from build123d import *

# Parameters (mm, degrees)
SKETCH_1_R               = 3.2
EXTRUDE_1_DEPTH          = 14
CUT_EXTRUDE_1_DEPTH      = 1
CUT_EXTRUDE_1_DEPTH_BACK = 10.4
SKETCH_3_W               = 0.65
SKETCH_3_H               = 3.2
CUT_EXTRUDE_2_DEPTH      = 1
SKETCH_4_W               = 0.4
SKETCH_4_H               = 2
EXTRUDE_2_DEPTH          = 4
EXTRUDE_2_2_DEPTH        = 4
SKETCH_4_W_2             = 2
SKETCH_4_H_2             = 0.4
EXTRUDE_2_3_DEPTH        = 4
EXTRUDE_3_DEPTH          = 2
EXTRUDE_4_DEPTH          = 2
SKETCH_8_R               = 3.2
SKETCH_8_R_2             = 0.603563731
EXTRUDE_5_DEPTH          = 2
SKETCH_9_R               = 0.5
CUT_EXTRUDE_3_DEPTH      = 10.8
SKETCH_10_R              = 0.5
CUT_EXTRUDE_4_DEPTH      = 2


with BuildPart() as part:
    # Sketch 1 → Extrude 1 (new body)
    with BuildSketch(Plane.XY):
        with BuildLine():
            Line((-4, 5.5), (4, 5.5))
            ThreePointArc((4, 5.5), (4.353553391, 5.353553391), (4.5, 5))
            Line((4.5, 5), (4.5, -5))
            ThreePointArc((4.5, -5), (4.353553391, -5.353553391), (4, -5.5))
            Line((4, -5.5), (-4, -5.5))
            ThreePointArc((-4, -5.5), (-4.353553391, -5.353553391), (-4.5, -5))
            Line((-4.5, -5), (-4.5, 5))
            ThreePointArc((-4.5, 5), (-4.353553391, 5.353553391), (-4, 5.5))
        make_face()
        with Locations((0, 1)):
            Circle(SKETCH_1_R, mode=Mode.SUBTRACT)
    extrude(amount=EXTRUDE_1_DEPTH)

    # Sketch 2 → Cut-Extrude 1 (cut, two sides)
    with BuildSketch(Plane.XY.offset(14)) as cut_extrude_1_sk:
        with BuildLine():
            ThreePointArc((-3.85, 1), (0, 4.85), (3.85, 1))
            Line((3.85, 1), (4.5, 1))
            Line((4.5, 1), (4.5, 5))
            ThreePointArc((4.5, 5), (4.353553391, 5.353553391), (4, 5.5))
            Line((4, 5.5), (-4, 5.5))
            ThreePointArc((-4, 5.5), (-4.353553391, 5.353553391), (-4.5, 5))
            Line((-4.5, 5), (-4.5, 1))
            Line((-4.5, 1), (-3.85, 1))
        make_face()
    extrude(amount=CUT_EXTRUDE_1_DEPTH, mode=Mode.SUBTRACT)
    extrude(cut_extrude_1_sk.sketch, amount=-CUT_EXTRUDE_1_DEPTH_BACK, mode=Mode.SUBTRACT)

    # Sketch 3 → Cut-Extrude 2 (cut)
    with BuildSketch(Plane.XY.offset(14)):
        with Locations((-4.175, -0.6)):
            Rectangle(SKETCH_3_W, SKETCH_3_H)
        with Locations((4.175, -0.6)):
            Rectangle(SKETCH_3_W, SKETCH_3_H)
    extrude(amount=-CUT_EXTRUDE_2_DEPTH, mode=Mode.SUBTRACT)



with BuildPart() as body_2:
    # Sketch 4 → Extrude 2 (new body)
    with BuildSketch(Plane(origin=(0, -5.5, 0), x_dir=(-1, 0, 0), z_dir=(0, -1, 0))):
        with Locations((4.7, -11)):
            Rectangle(SKETCH_4_W, SKETCH_4_H)
    extrude(amount=EXTRUDE_2_DEPTH)


with BuildPart() as body_3:
    # Sketch 4 → Extrude 2 2 (new body)
    with BuildSketch(Plane(origin=(0, -5.5, 0), x_dir=(-1, 0, 0), z_dir=(0, -1, 0))):
        with Locations((-4.7, -11)):
            Rectangle(SKETCH_4_W, SKETCH_4_H)
    extrude(amount=EXTRUDE_2_2_DEPTH)


with BuildPart() as body_4:
    # Sketch 4 → Extrude 2 3 (new body)
    with BuildSketch(Plane(origin=(0, -5.5, 0), x_dir=(-1, 0, 0), z_dir=(0, -1, 0))):
        with Locations((0, -13.7)):
            Rectangle(SKETCH_4_W_2, SKETCH_4_H_2)
    extrude(amount=EXTRUDE_2_3_DEPTH)


with BuildPart() as part_1:
    add(part.part)

    add(body_2.part)  # Extrude 3 merges body 2

    add(body_3.part)  # Extrude 3 merges body 3
    # Sketch 5 → Extrude 3 (add)
    with BuildSketch(Plane(origin=(0, 0, 10), x_dir=(-1, 0, 0), z_dir=(0, 0, -1))):
        with BuildLine():
            Line((4.5, -5.5), (4.5, -1.092241159))
            Line((4.5, -1.092241159), (4.6, -1.092241159))
            ThreePointArc((4.6, -1.092241159), (4.812132034, -1.180109124), (4.9, -1.392241159))
            Line((4.9, -1.392241159), (4.9, -5.5))
            Line((4.9, -5.5), (4.5, -5.5))
        make_face()
        with BuildLine():
            Line((-4.9, -1.392241159), (-4.9, -5.5))
            Line((-4.9, -5.5), (-4.5, -5.5))
            Line((-4.5, -5.5), (-4.5, -1.092241159))
            Line((-4.5, -1.092241159), (-4.6, -1.092241159))
            ThreePointArc((-4.6, -1.092241159), (-4.812132034, -1.180109124), (-4.9, -1.392241159))
        make_face()
    extrude(amount=-EXTRUDE_3_DEPTH)


    add(body_4.part)  # Extrude 4 merges body 4
    # Sketch 7 → Extrude 4 (add)
    with BuildSketch(Plane.ZY.offset(1)):
        with BuildLine():
            Line((14, -5.5), (14, 1))
            Line((14, 1), (13.6, 1))
            ThreePointArc((13.6, 1), (13.812132034, 0.912132034), (13.9, 0.7))
            Line((13.9, 0.7), (13.9, -5.5))
            Line((13.9, -5.5), (14, -5.5))
        make_face()
    extrude(amount=-EXTRUDE_4_DEPTH)

    # Sketch 8 → Extrude 5 (add)
    with BuildSketch(Plane.XY.offset(14)):
        with Locations((0, 1)):
            Circle(SKETCH_8_R)
        with Locations((0, 1)):
            Circle(SKETCH_8_R_2, mode=Mode.SUBTRACT)
    extrude(amount=-EXTRUDE_5_DEPTH)

    # Sketch 9 → Cut-Extrude 3 (cut, through all)
    with BuildSketch(Plane.ZY.offset(4.9)):
        with Locations((11, -8.5)):
            Circle(SKETCH_9_R)
        with BuildLine():
            Line((10, -8.5), (10, -9.805302044))
            Line((10, -9.805302044), (12, -9.805302044))
            Line((12, -9.805302044), (12, -8.5))
            ThreePointArc((12, -8.5), (11, -9.5), (10, -8.5))
        make_face()
    extrude(amount=-CUT_EXTRUDE_3_DEPTH, mode=Mode.SUBTRACT)

    # Sketch 10 → Cut-Extrude 4 (cut)
    with BuildSketch(Plane.XY.offset(13.9)):
        with Locations((0, -8.5)):
            Circle(SKETCH_10_R)
        with BuildLine():
            Line((-1, -8.5), (-1, -10.359825608))
            Line((-1, -10.359825608), (1, -10.359825608))
            Line((1, -10.359825608), (1, -8.5))
            ThreePointArc((1, -8.5), (0, -9.5), (-1, -8.5))
        make_face()
    extrude(amount=-CUT_EXTRUDE_4_DEPTH, mode=Mode.SUBTRACT)


solid = part_1.part
Here's how the part is built. I have some questions about the finished solid (model axes, mm). A direction names the side the tool comes from. Coordinates: 2 decimals unless noted, no trailing zeros. Loops run counter-clockwise (first coordinate to the right, second up) from the corner with the lowest first, then second, coordinate; pieces in that order, holes last. Notation, with made-up numbers: (69, 29) -> (73, 29) arc R21 ccw to (73, 51) -> close; hole circle Ø1 at (52.25, -32). An arc over 180 degrees is marked (long way). Use one line per item in the form item = value. Start each with the question number.
(1) Please list where these lines run through material, in increasing order: line 1 along X through (y, z) = (1, 13.15); line 2 along Y through (x, z) = (4.6, 11); line 3 along Z through (x, y) = (0, -0.25).
(2) Will these pins go through, and if not, where does the flat tip stop? pin 1 (0.5 mm diameter, centred on x = 4.5, z = 13.5, fed in from +Y); pin 2 (2 mm diameter, centred on x = 0.5, y = -7.5, fed in from +Z); pin 3 (2.5 mm diameter, centred on x = -1.5, z = 4, fed in from -Y).
(3) We'd pull the mould along Z, two halves only. Please class faces 5 (the face through (-4.703, -8.988, 10.892)), 6 (the face through (-0.08, 4.85, 8.87)), 7 (the face through (0, 0, 12)), 8 (the face through (4.697, -8.988, 10.892)): pulls with the +Z half, pulls with the -Z half, needs draft (parallel to the pull), parting line crosses it, or undercut.
(4) If we section it at C-C (z = 2.25): Please give me the cut outline in (x, y), then the cut area to 3 significant figures.
(5) On a 3-axis mill with a long thin cutter (end or side, diameter ignored), from which of +Z, -Z, +X, -X, +Y, -Y can I reach the whole of each face in a straight line? I mean faces 1 (the face through (0, -7, 13.5)), 2 (the face through (-3.85, -0.6, 13.5)), 3 (the face through (-0.694, -2.124, 5.916)), 4 (the face through (0, -7, 13.9)). Say none if no direction works.
(6) If we section it at A-A (z = 11): Please give me the cut outline in (x, y), then the cut area to 3 significant figures.
(7) If we section it at B-B (x = 0): Please give me the cut outline in (y, z).
(8) If we section it at D-D (y = -0.5): Please give me the cut outline in (x, z), then the cut area to 3 significant figures.
Verdict:
q1.line_1 = -3.85 to -0.6, 0.6 to 3.85
q1.line_2 = -9.5 to -9, -8 to -1.09
q1.line_3 = 12 to 14
q2.pin_1 = -2.2
q2.pin_2 = 13.9
q2.pin_3 = -5.5
q3.face_5 = undercut
q3.face_6 = needs draft
q3.face_7 = pulls with the -Z half
q3.face_8 = undercut
q4.outline = (-4.5, -5) arc R0.5 ccw to (-4, -5.5) -> (4, -5.5) arc R0.5 ccw to (4.5, -5) -> (4.5, 5) arc R0.5 ccw to (4, 5.5) -> (-4, 5.5) arc R0.5 ccw to (-4.5, 5) -> close; hole circle Ø6.4 at (0, 1)
q4.area = 66.6 mm²
q5.face_1 = -Z, +X, -X, -Y
q5.face_2 = +Z, -X, +Y
q5.face_3 = -Z
q5.face_4 = +Z, +X, -X, -Y
q6.outline = (-4.9, -9.5) -> (-4.5, -9.5) -> (-4.5, -9) -> (-4.9, -9) -> close; (-4.9, -8) -> (-4.5, -8) -> (-4.5, -5) arc R0.5 ccw to (-4, -5.5) -> (4, -5.5) arc R0.5 ccw to (4.5, -5) -> (4.5, -8) -> (4.9, -8) -> (4.9, -1.39) arc R0.3 ccw to (4.6, -1.09) -> (4.5, -1.09) -> (4.5, 1) -> (3.85, 1) arc R3.85 ccw to (-3.85, 1) -> (-4.5, 1) -> (-4.5, -1.09) -> (-4.6, -1.09) arc R0.3 ccw to (-4.9, -1.39) -> close; (4.5, -9.5) -> (4.9, -9.5) -> (4.9, -9) -> (4.5, -9) -> close; hole circle Ø6.4 at (0, 1)
q6.area = 55.4 mm²
q7.outline = (-9.5, 13.5) -> (-9, 13.5) -> (-9, 13.9) -> (-9.5, 13.9) -> close; (-8, 13.5) -> (-5.5, 13.5) -> (-5.5, 0) -> (-2.2, 0) -> (-2.2, 12) -> (0.4, 12) -> (0.4, 13.9) -> (0.7, 13.9) arc R0.3 cw to (1, 13.6) -> (1, 14) -> (-5.5, 14) -> (-5.5, 13.9) -> (-8, 13.9) -> close; (1.6, 12) -> (4.2, 12) -> (4.2, 0) -> (5.5, 0) -> (5.5, 3.6) -> (4.85, 3.6) -> (4.85, 14) -> (1.6, 14) -> close
q8.outline = (-4.5, 0) -> (-2.83, 0) -> (-2.83, 12) -> (2.83, 12) -> (2.83, 0) -> (4.5, 0) -> (4.5, 13) -> (3.85, 13) -> (3.85, 14) -> (-3.85, 14) -> (-3.85, 13) -> (-4.5, 13) -> close
q8.area = 56.9 mm²
